Geometry: final body of the model. Coordinates: model frame, mm. Face numbers are marked on the shaded views. A direction names the side the tool comes from. Give positions to 0.01 mm unless a question says otherwise; leave off trailing zeros. Loops run counter-clockwise (first coordinate to the right, second up) from the corner with the lowest first, then second, coordinate; pieces in that order, holes last. Notation, with made-up numbers: M 28.25,-22 L 77.25,-22 A20 cw 77.25,-15 Z; hole C -40,-36.5 d10. An arc over 180 degrees is marked long. Put each result on its own line as item: value.
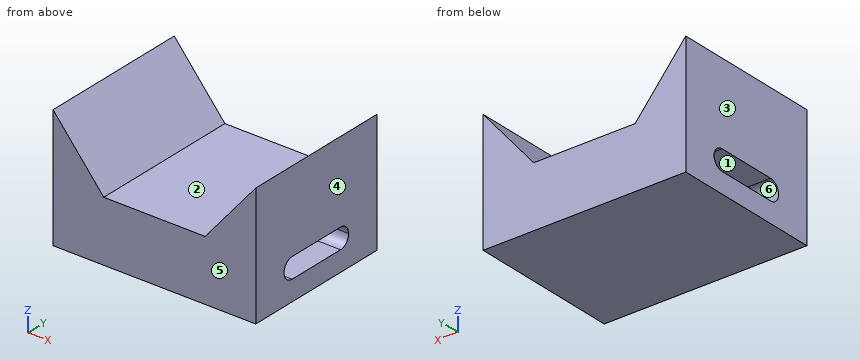
```python
from build123d import *

# Parameters (mm, degrees)
F1_DEPTH = 75
F3_DEPTH = 200.001


with BuildPart() as f1:
    # F0 (on Front) → F1 (new body, symmetric)
    with BuildSketch(Plane.XZ):
        Polygon((-100, -60), (100, -60), (100, 60), (50, 0), (-50, 0), (-100, 60), align=None)
    extrude(amount=F1_DEPTH, both=True)

    # F2 (on face) → F3 (cut, through all)
    with BuildSketch(Plane.YZ.offset(100)):
        with BuildLine():
            ThreePointArc((30, -40), (20, -30), (30, -20))
            Line((30, -20), (-30, -20))
            ThreePointArc((-30, -20), (-22.9289321881, -22.9289321881), (-20, -30))
            ThreePointArc((-20, -30), (-22.9289321881, -37.0710678119), (-30, -40))
            Line((-30, -40), (30, -40))
        make_face()
        with BuildLine():
            ThreePointArc((40, -30), (37.0710678119, -22.9289321881), (30, -20))
            Line((30, -20), (30, -40))
            ThreePointArc((30, -40), (37.0710678119, -37.0710678119), (40, -30))
        make_face()
        with BuildLine():
            Line((30, -40), (30, -20))
            ThreePointArc((30, -20), (20, -30), (30, -40))
        make_face()
        with BuildLine():
            ThreePointArc((-20, -30), (-22.9289321881, -22.9289321881), (-30, -20))
            Line((-30, -20), (-30, -40))
            ThreePointArc((-30, -40), (-22.9289321881, -37.0710678119), (-20, -30))
        make_face()
        with BuildLine():
            Line((-30, -40), (-30, -20))
            ThreePointArc((-30, -20), (-40, -30), (-30, -40))
        make_face()
    extrude(amount=-F3_DEPTH, mode=Mode.SUBTRACT)


solid = f1.part
```
Item 1: Section B-B on z = 36. Output: boundary loops of the cut face in (x, y).
Output values:
outline: M -100,-75 L -80,-75 L -80,75 L -100,75 Z; M 80,-75 L 100,-75 L 100,75 L 80,75 Z
Item 2: Line query: probe 1 along Z at (x, y) = (26, 5.5); probe 2 along Z at (x, y) = (35.5, 39); probe 3 along Y at (x, z) = (62.5, -31). Output: solid intervals per line, ascending. Write a range as [from, to].
Output values:
probe 1: [-60, -40], [-20, 0]
probe 2: [-60, -34.36], [-25.64, 0]
probe 3: [-75, -39.95], [39.95, 75]
Item 3: Pin query (flat end, axial travel): pin 1 Ø1 at (x, y) = (-18, -42) entering from +Z. Return the tip coordinate at first contact, or that it passes through.
Output values:
pin 1: z = 0
Item 4: Section D-D on y = 44.5. Output: boundary loops of the cut face in (x, z).
Output values:
outline: M -100,-60 L 100,-60 L 100,60 L 50,0 L -50,0 L -100,60 Z
Item 5: Section C-C on x = 74.5. Output: boundary loops of the cut face in (y, z).
Output values:
outline: M -75,-60 L 75,-60 L 75,29.4 L -75,29.4 Z; hole M -30,-40 L 30,-40 A10 ccw 30,-20 L -30,-20 A10 ccw Z
Item 6: Section A-A on y = 8.5. Output: boundary loops of the cut face in (x, z).
Output values:
outline: M -100,-60 L 100,-60 L 100,-40 L -100,-40 Z; M -100,-20 L 100,-20 L 100,60 L 50,0 L -50,0 L -100,60 Z
Item 7: Mould query, pull axis Y, two halves, no side actions, for the marked faces 4, 5 and 6. Classes: pulls with the +Y half, pulls with the -Y half, needs draft (parallel to the pull), parting line crosses it, or undercut.
Output values:
face 4: needs draft
face 5: pulls with the -Y half
face 6: undercut
Item 8: Set-up query: the marked faces 1, 2 and 3. Return all of +Z, -Z, +X, -X, +Y, -Y with unobstructed straight access to the full face (end or side cutting, diameter ignored); none if empty.
Output values:
face 1: +X, -X
face 2: +Z, +Y, -Y
face 3: +Z, -Z, -X, +Y, -Y
